from build123d import *

# Parameters (mm, degrees)
SKETCH1_W           = 11
SKETCH1_H           = 72
BOSS_EXTRUDE1_DEPTH = 12
SKETCH2_W           = 12
SKETCH2_H           = 10
SKETCH2_R           = 1.5
BOSS_EXTRUDE2_DEPTH = 2
SKETCH3_W           = 7
SKETCH3_H           = 7
CUT_EXTRUDE1_DEPTH  = 3
SKETCH4_W           = 7
SKETCH4_H           = 69
CUT_EXTRUDE2_DEPTH  = 10.5
CUT_EXTRUDE3_DEPTH  = 1.5


with BuildPart() as part:
    # Sketch1 → Boss-Extrude1 (new body)
    with BuildSketch(Plane.XY):
        with Locations((5.5, 36)):
            Rectangle(SKETCH1_W, SKETCH1_H)
    extrude(amount=BOSS_EXTRUDE1_DEPTH)

    # Sketch2 → Boss-Extrude2 (add)
    # profile 1 of 2: a face of its own
    with BuildSketch(Plane(origin=(11, 0, 0), x_dir=(0, 0, -1), z_dir=(1, 0, 0))):
        with Locations((-6, 77)):
            Rectangle(SKETCH2_W, SKETCH2_H)
        with Locations((-6, 77)):
            Circle(SKETCH2_R, mode=Mode.SUBTRACT)
    # profile 2 of 2: a face of its own
    with BuildSketch(Plane(origin=(11, 0, 0), x_dir=(0, 0, -1), z_dir=(1, 0, 0))):
        with Locations((-6, -5)):
            Rectangle(SKETCH2_W, SKETCH2_H)
        with Locations(Location((-6, -5, 0), (0, 0, 180))):
            Circle(SKETCH2_R, mode=Mode.SUBTRACT)
    extrude(amount=-BOSS_EXTRUDE2_DEPTH)

    # Sketch3 → Cut-Extrude1 (cut)
    with BuildSketch(Plane(origin=(11, 0, 0), x_dir=(0, 0, -1), z_dir=(1, 0, 0))):
        with Locations((-6, 65.5)):
            Rectangle(SKETCH3_W, SKETCH3_H)
        with Locations((-6, 6.5)):
            Rectangle(SKETCH3_W, SKETCH3_H)
    extrude(amount=-CUT_EXTRUDE1_DEPTH, mode=Mode.SUBTRACT)

    # Sketch4 → Cut-Extrude2 (cut)
    with BuildSketch(Plane.XY.offset(12)):
        with Locations((5, 36)):
            Rectangle(SKETCH4_W, SKETCH4_H)
    extrude(amount=-CUT_EXTRUDE2_DEPTH, mode=Mode.SUBTRACT)

    # Sketch5 → Cut-Extrude3 (cut)
    with BuildSketch(Plane.ZY):
        with BuildLine():
            Line((6.25, 66), (9.75, 66))
            ThreePointArc((9.75, 66), (10.280330086, 65.780330086), (10.5, 65.25))
            Line((10.5, 65.25), (10.5, 64.75))
            ThreePointArc((10.5, 64.75), (10.280330086, 64.219669914), (9.75, 64))
            Line((9.75, 64), (6.25, 64))
            ThreePointArc((6.25, 64), (5.719669914, 64.219669914), (5.5, 64.75))
            Line((5.5, 64.75), (5.5, 65.25))
            ThreePointArc((5.5, 65.25), (5.719669914, 65.780330086), (6.25, 66))
        make_face()
        with BuildLine():
            Line((6.25, 8), (9.75, 8))
            ThreePointArc((9.75, 8), (10.280330086, 7.780330086), (10.5, 7.25))
            Line((10.5, 7.25), (10.5, 6.75))
            ThreePointArc((10.5, 6.75), (10.280330086, 6.219669914), (9.75, 6))
            Line((9.75, 6), (6.25, 6))
            ThreePointArc((6.25, 6), (5.719669914, 6.219669914), (5.5, 6.75))
            Line((5.5, 6.75), (5.5, 7.25))
            ThreePointArc((5.5, 7.25), (5.719669914, 7.780330086), (6.25, 8))
        make_face()
    extrude(amount=-CUT_EXTRUDE3_DEPTH, mode=Mode.SUBTRACT)


solid = part.part
Build history of the part. All positions in model axes, mm. A direction names the side the tool comes from. Give positions to 0.01 mm unless a question says otherwise; leave off trailing zeros. Order: outer loops, then holes, each group sorted by start corner. A loop starts at its lowest first (then second) coordinate and runs counter-clockwise, first axis right, second up. Notation, with made-up numbers: M 81,27 L 114,27 A26 cw 114,42 Z; hole C 41.25,-37.5 d7. An arc over 180 degrees is marked long. Use one line per item in the form item = value.
1) Saw through at B-B (y = -5). Give the cut face in (x, z), plus the area to 3 significant figures.
Calculated:
outline = M 9,0 L 11,0 L 11,4.5 L 9,4.5 Z; M 9,7.5 L 11,7.5 L 11,12 L 9,12 Z
area = 18.0 mm2
2) Saw through at A-A (z = 3.5). Give the cut face in (x, y).
Calculated:
outline = M 0,0 L 9,0 L 9,-10 L 11,-10 L 11,3 L 8.5,3 L 8.5,1.5 L 1.5,1.5 L 1.5,70.5 L 8.5,70.5 L 8.5,69 L 11,69 L 11,82 L 9,82 L 9,72 L 0,72 Z; M 8.5,10 L 11,10 L 11,62 L 8.5,62 Z
3) Saw through at D-D (y = 31). Give the cut face in (x, z), plus the area to 3 significant figures.
Calculated:
outline = M 0,0 L 11,0 L 11,12 L 8.5,12 L 8.5,1.5 L 1.5,1.5 L 1.5,12 L 0,12 Z
area = 58.5 mm2
4) Tool access for faces 1 (the face through (5, 1.5, 7)), 2 (the face through (10, 65, 2.5)), 3 (the face through (4, 0, 6)), 4 (the face through (4, 72, 6)): list every direction of +Z, -Z, +X, -X, +Y, -Y with a clear straight run to the whole face (end or side of a thin tool).
Calculated:
face_1 = +Z
face_2 = +X
face_3 = +Z, -Z, -X, -Y
face_4 = +Z, -Z, -X, +Y
5) Probe probe 1 along Y at (x, z) = (10.35, 6); probe 2 along Y at (x, z) = (10.25, 2.75); probe 3 along Z at (x, y) = (10.15, -5). List the from-to ranges inside material, lowest first.
Calculated:
probe_1 = -10 to -6.5, -3.5 to 3, 10 to 62, 69 to 75.5, 78.5 to 82
probe_2 = -10 to 3, 10 to 62, 69 to 82
probe_3 = 0 to 4.5, 7.5 to 12
6) Drop flat-ended pins along their axis: pin 1 (5.5 mm diameter, centred on x = 4, z = 8.5, fed in from +Y); pin 2 (3 mm diameter, centred on y = -5.5, z = 4, fed in from -X). Give the stop position or say it passes through.
Calculated:
pin_1 = 72
pin_2 = 9
7) Saw through at C-C (x = 6.5). Give the cut face in (y, z), plus the area to 4 significant figures.
Calculated:
outline = M 0,0 L 72,0 L 72,12 L 70.5,12 L 70.5,1.5 L 1.5,1.5 L 1.5,12 L 0,12 Z
area = 139.5 mm2
8) Two-plate mould, pull along X, no slides. Class faces 5 (the face through (10, 6, 9.5)), 6 (the face through (11, 37, 6)), 7 (the face through (5, 70.5, 7)): released by +X, released by -X, zero draft, split by the parting line, or undercut.
Calculated:
face_5 = zero draft
face_6 = released by +X
face_7 = undercut
